```python
from build123d import *

# Parameters (mm, degrees)
SKETCH1_W           = 19
SKETCH1_H           = 27
BOSS_EXTRUDE1_DEPTH = 2
SKETCH2_W           = 19
SKETCH2_H           = 2
BOSS_EXTRUDE2_DEPTH = 40
BOSS_EXTRUDE3_DEPTH = 2
SKETCH5_W           = 6
SKETCH5_H           = 2
BOSS_EXTRUDE4_DEPTH = 25
SKETCH6_R           = 1.5
CUT_EXTRUDE1_DEPTH  = 2
CUT_EXTRUDE2_REACH  = 9
SKETCH7_R           = 1.5
CUT_EXTRUDE4_REACH  = 29
SKETCH9_R           = 1.5


with BuildPart() as part:
    # Sketch1 → Boss-Extrude1 (new body)
    with BuildSketch(Plane.XY):
        with Locations((9.5, 13.5)):
            Rectangle(SKETCH1_W, SKETCH1_H)
    boss_extrude1 = extrude(amount=BOSS_EXTRUDE1_DEPTH)

    # Sketch2 → Boss-Extrude2 (add)
    with BuildSketch(Plane.XY.offset(2)):
        with Locations((9.5, 26)):
            Rectangle(SKETCH2_W, SKETCH2_H)
    boss_extrude2 = extrude(amount=BOSS_EXTRUDE2_DEPTH)

    # Sketch3 → Boss-Extrude3 (add)
    with BuildSketch(Plane(origin=(0, 25, 0), x_dir=(-1, 0, 0), z_dir=(0, -1, 0))):
        Polygon((-19, -32), (-19, -9), (-27, -9), (-27, -37), (-21, -37), (-21, -32), align=None)
    boss_extrude3 = extrude(amount=-BOSS_EXTRUDE3_DEPTH)

    # Sketch5 → Boss-Extrude4 (add)
    with BuildSketch(Plane(origin=(0, 25, 0), x_dir=(-1, 0, 0), z_dir=(0, -1, 0))):
        with Locations((-24, -36)):
            Rectangle(SKETCH5_W, SKETCH5_H)
    boss_extrude4 = extrude(amount=BOSS_EXTRUDE4_DEPTH)

    # Sketch6 → Cut-Extrude1 (cut)
    with BuildSketch(Plane.XY.offset(2)):
        with Locations((12, 3)):
            Circle(SKETCH6_R)
        with Locations((12, 10)):
            Circle(SKETCH6_R)
        with Locations((12, 17)):
            Circle(SKETCH6_R)
        with Locations((5, 10)):
            Circle(SKETCH6_R)
    cut_extrude1 = extrude(amount=-CUT_EXTRUDE1_DEPTH, mode=Mode.SUBTRACT)

    # Mirror2: Boss-Extrude1, Boss-Extrude2, Boss-Extrude3, Boss-Extrude4, Cut-Extrude1 across plane
    add(boss_extrude1.mirror(Plane(origin=(0, 0, 2), x_dir=(0, 0, 1), z_dir=(1, 0, 0))))
    add(boss_extrude2.mirror(Plane(origin=(0, 0, 2), x_dir=(0, 0, 1), z_dir=(1, 0, 0))))
    add(boss_extrude3.mirror(Plane(origin=(0, 0, 2), x_dir=(0, 0, 1), z_dir=(1, 0, 0))))
    add(boss_extrude4.mirror(Plane(origin=(0, 0, 2), x_dir=(0, 0, 1), z_dir=(1, 0, 0))))
    add(cut_extrude1.mirror(Plane(origin=(0, 0, 2), x_dir=(0, 0, 1), z_dir=(1, 0, 0))), mode=Mode.SUBTRACT)

    # Sketch7 → Cut-Extrude2 (cut, up to next)
    with BuildSketch(Plane(origin=(0, 0, 35), x_dir=(-1, 0, 0), z_dir=(0, 0, -1)), mode=Mode.PRIVATE) as cut_extrude2_sk1:
        with Locations((-23.456279898, 5.5)):
            Circle(SKETCH7_R)
    cut_extrude2_tool1 = extrude(cut_extrude2_sk1.sketch, amount=-CUT_EXTRUDE2_REACH, mode=Mode.PRIVATE) & part.part
    add(cut_extrude2_tool1.solids().sort_by_distance((23.45628, 5.5, 35))[0], mode=Mode.SUBTRACT)
    # Sketch7 → Cut-Extrude2 (cut, up to next)
    with BuildSketch(Plane(origin=(0, 0, 35), x_dir=(-1, 0, 0), z_dir=(0, 0, -1)), mode=Mode.PRIVATE) as cut_extrude2_sk2:
        with Locations((-23.456279898, 14.5)):
            Circle(SKETCH7_R)
    cut_extrude2_tool2 = extrude(cut_extrude2_sk2.sketch, amount=-CUT_EXTRUDE2_REACH, mode=Mode.PRIVATE) & part.part
    add(cut_extrude2_tool2.solids().sort_by_distance((23.45628, 14.5, 35))[0], mode=Mode.SUBTRACT)
    # Sketch7 → Cut-Extrude2 (cut, up to next)
    with BuildSketch(Plane(origin=(0, 0, 35), x_dir=(-1, 0, 0), z_dir=(0, 0, -1)), mode=Mode.PRIVATE) as cut_extrude2_sk3:
        with Locations((23.543720102, 5.5)):
            Circle(SKETCH7_R)
    cut_extrude2_tool3 = extrude(cut_extrude2_sk3.sketch, amount=-CUT_EXTRUDE2_REACH, mode=Mode.PRIVATE) & part.part
    add(cut_extrude2_tool3.solids().sort_by_distance((-23.54372, 5.5, 35))[0], mode=Mode.SUBTRACT)
    # Sketch7 → Cut-Extrude2 (cut, up to next)
    with BuildSketch(Plane(origin=(0, 0, 35), x_dir=(-1, 0, 0), z_dir=(0, 0, -1)), mode=Mode.PRIVATE) as cut_extrude2_sk4:
        with Locations((23.543720102, 14.5)):
            Circle(SKETCH7_R)
    cut_extrude2_tool4 = extrude(cut_extrude2_sk4.sketch, amount=-CUT_EXTRUDE2_REACH, mode=Mode.PRIVATE) & part.part
    add(cut_extrude2_tool4.solids().sort_by_distance((-23.54372, 14.5, 35))[0], mode=Mode.SUBTRACT)

    # Sketch9 → Cut-Extrude4 (cut, up to next)
    with BuildSketch(Plane(origin=(0, 27, 0), x_dir=(1, 0, 0), z_dir=(0, 1, 0)), mode=Mode.PRIVATE) as cut_extrude4_sk1:
        with Locations((12, -32)):
            Circle(SKETCH9_R)
    cut_extrude4_tool1 = extrude(cut_extrude4_sk1.sketch, amount=-CUT_EXTRUDE4_REACH, mode=Mode.PRIVATE) & part.part
    add(cut_extrude4_tool1.solids().sort_by_distance((12, 27, 32))[0], mode=Mode.SUBTRACT)
    # Sketch9 → Cut-Extrude4 (cut, up to next)
    with BuildSketch(Plane(origin=(0, 27, 0), x_dir=(1, 0, 0), z_dir=(0, 1, 0)), mode=Mode.PRIVATE) as cut_extrude4_sk2:
        with Locations((12, -25)):
            Circle(SKETCH9_R)
    cut_extrude4_tool2 = extrude(cut_extrude4_sk2.sketch, amount=-CUT_EXTRUDE4_REACH, mode=Mode.PRIVATE) & part.part
    add(cut_extrude4_tool2.solids().sort_by_distance((12, 27, 25))[0], mode=Mode.SUBTRACT)
    # Sketch9 → Cut-Extrude4 (cut, up to next)
    with BuildSketch(Plane(origin=(0, 27, 0), x_dir=(1, 0, 0), z_dir=(0, 1, 0)), mode=Mode.PRIVATE) as cut_extrude4_sk3:
        with Locations((12, -39)):
            Circle(SKETCH9_R)
    cut_extrude4_tool3 = extrude(cut_extrude4_sk3.sketch, amount=-CUT_EXTRUDE4_REACH, mode=Mode.PRIVATE) & part.part
    add(cut_extrude4_tool3.solids().sort_by_distance((12, 27, 39))[0], mode=Mode.SUBTRACT)
    # Sketch9 → Cut-Extrude4 (cut, up to next)
    with BuildSketch(Plane(origin=(0, 27, 0), x_dir=(1, 0, 0), z_dir=(0, 1, 0)), mode=Mode.PRIVATE) as cut_extrude4_sk4:
        with Locations((5, -32)):
            Circle(SKETCH9_R)
    cut_extrude4_tool4 = extrude(cut_extrude4_sk4.sketch, amount=-CUT_EXTRUDE4_REACH, mode=Mode.PRIVATE) & part.part
    add(cut_extrude4_tool4.solids().sort_by_distance((5, 27, 32))[0], mode=Mode.SUBTRACT)
    # Sketch9 → Cut-Extrude4 (cut, up to next)
    with BuildSketch(Plane(origin=(0, 27, 0), x_dir=(1, 0, 0), z_dir=(0, 1, 0)), mode=Mode.PRIVATE) as cut_extrude4_sk5:
        with Locations((-5, -32)):
            Circle(SKETCH9_R)
    cut_extrude4_tool5 = extrude(cut_extrude4_sk5.sketch, amount=-CUT_EXTRUDE4_REACH, mode=Mode.PRIVATE) & part.part
    add(cut_extrude4_tool5.solids().sort_by_distance((-5, 27, 32))[0], mode=Mode.SUBTRACT)
    # Sketch9 → Cut-Extrude4 (cut, up to next)
    with BuildSketch(Plane(origin=(0, 27, 0), x_dir=(1, 0, 0), z_dir=(0, 1, 0)), mode=Mode.PRIVATE) as cut_extrude4_sk6:
        with Locations((-12, -32)):
            Circle(SKETCH9_R)
    cut_extrude4_tool6 = extrude(cut_extrude4_sk6.sketch, amount=-CUT_EXTRUDE4_REACH, mode=Mode.PRIVATE) & part.part
    add(cut_extrude4_tool6.solids().sort_by_distance((-12, 27, 32))[0], mode=Mode.SUBTRACT)
    # Sketch9 → Cut-Extrude4 (cut, up to next)
    with BuildSketch(Plane(origin=(0, 27, 0), x_dir=(1, 0, 0), z_dir=(0, 1, 0)), mode=Mode.PRIVATE) as cut_extrude4_sk7:
        with Locations((-12, -39)):
            Circle(SKETCH9_R)
    cut_extrude4_tool7 = extrude(cut_extrude4_sk7.sketch, amount=-CUT_EXTRUDE4_REACH, mode=Mode.PRIVATE) & part.part
    add(cut_extrude4_tool7.solids().sort_by_distance((-12, 27, 39))[0], mode=Mode.SUBTRACT)
    # Sketch9 → Cut-Extrude4 (cut, up to next)
    with BuildSketch(Plane(origin=(0, 27, 0), x_dir=(1, 0, 0), z_dir=(0, 1, 0)), mode=Mode.PRIVATE) as cut_extrude4_sk8:
        with Locations((-12, -25)):
            Circle(SKETCH9_R)
    cut_extrude4_tool8 = extrude(cut_extrude4_sk8.sketch, amount=-CUT_EXTRUDE4_REACH, mode=Mode.PRIVATE) & part.part
    add(cut_extrude4_tool8.solids().sort_by_distance((-12, 27, 25))[0], mode=Mode.SUBTRACT)


solid = part.part
```
Input: part model. Units: mm. Frame: model coordinates. A direction names the side the tool comes from. Give positions to 0.01 mm unless a question says otherwise; leave off trailing zeros. Order: outer loops, then holes, each group sorted by start corner. A loop starts at its lowest first (then second) coordinate and runs counter-clockwise, first axis right, second up. Notation, with made-up numbers: (58, 31.5) -> (91, 31.5) arc R23 cw to (91, 40.5) -> close; hole circle Ø7 at (-1.5, -37). An arc over 180 degrees is marked (long way). Write each question's results on one line, items separated by ' | '. Start each with the question number.
Item 1: Line query: line 1 (Z direction, x = -12, y = 26.1); line 2 (Y direction, x = -12, z = 1.15); line 3 (Y direction, x = 9, z = 10). Output: solid intervals per line, ascending.
Item 2: Cut plane C-C on x = -12. Give the number of separate pieces and of enclosed holes in the cut face, then the cut area to 3 significant figures.
Item 3: Contact query for flat-ended pins moving along their axis: P1, Ø2, axis at x = 21.5, y = 6.5, coming from the -Z side; P2, Ø5, axis at x = -12, z = 32, coming from the -Y side; P3, Ø4, axis at x = 5, y = 10, coming from the +Z side. Output: stop coordinate, or through.
Item 4: Mould query, pull axis Z, two halves, no side actions, for faces 1 (the cylindrical face through (10.8, 26, 32.9)), 2 (the cylindrical face through (-6.386, 9.425, 1.014)), 3 (the cylindrical face through (-12.325, 26.014, 40.464)), 4 (the flat face through (25.4, 13.7, 37)). Classes: pulls with the +Z half, pulls with the -Z half, needs draft (parallel to the pull), parting line crosses it, or undercut.
Item 5: Cut plane D-D on x = 5. Return the cut outline in (y, z), then the cut area to 3 significant figures.
Item 6: Set-up query: faces 5 (the flat face through (19, 15, 1)), 6 (the flat face through (0, 13, 2)), 7 (the flat face through (21, 14, 36)). Return all of +Z, -Z, +X, -X, +Y, -Y with unobstructed straight access to the full face (end or side cutting, diameter ignored); none if empty.
Item 7: Cut plane B-B on y = 10. Return the cut outline in (x, z), then the cut area to 3 significant figures.
Item 8: Cut plane A-A on y = 21. Return the cut outline in (x, z), then the cut area to 3 significant figures.
Established:
1) line 1: 0 to 23.5, 26.5 to 30.5, 33.5 to 37.5, 40.5 to 42 | line 2: 0 to 1.5, 4.5 to 8.5, 11.5 to 15.5, 18.5 to 27 | line 3: 25 to 27
2) separate pieces: 7 | enclosed holes: 0 | area: 98.0 mm^2
3) P1: z = 35 | P2: y = 25 | P3: z = 2
4) face 1: undercut | face 2: needs draft | face 3: undercut | face 4: pulls with the +Z half
5) outline: (0, 0) -> (8.5, 0) -> (8.5, 2) -> (0, 2) -> close; (11.5, 0) -> (27, 0) -> (27, 30.5) -> (25, 30.5) -> (25, 2) -> (11.5, 2) -> close; (25, 33.5) -> (27, 33.5) -> (27, 42) -> (25, 42) -> close | area: 122 mm^2
6) face 5: -Z, +X, +Y, -Y | face 6: +Z, +X, -X, -Y | face 7: +Z, +Y, -Y
7) outline: (-27, 35) -> (-21, 35) -> (-21, 37) -> (-27, 37) -> close; (-19, 0) -> (-13.5, 0) -> (-13.5, 2) -> (-19, 2) -> close; (-10.5, 0) -> (-6.5, 0) -> (-6.5, 2) -> (-10.5, 2) -> close; (-3.5, 0) -> (3.5, 0) -> (3.5, 2) -> (-3.5, 2) -> close; (6.5, 0) -> (10.5, 0) -> (10.5, 2) -> (6.5, 2) -> close; (13.5, 0) -> (19, 0) -> (19, 2) -> (13.5, 2) -> close; (21, 35) -> (27, 35) -> (27, 37) -> (21, 37) -> close | area: 76.0 mm^2
8) outline: (-27, 35) -> (-21, 35) -> (-21, 37) -> (-27, 37) -> close; (-19, 0) -> (19, 0) -> (19, 2) -> (-19, 2) -> close; (21, 35) -> (27, 35) -> (27, 37) -> (21, 37) -> close | area: 100 mm^2
